```python
from build123d import *

# Parameters (mm, degrees)
EXTRUDE_1_DEPTH     = 1.45
SKETCH_3_R          = 3.5
EXTRUDE_2_DEPTH     = 2.02
SKETCH_4_R          = 2
CUT_EXTRUDE_1_DEPTH = 8.265654364
EXTRUDE_START       = -0.2
SKETCH_5_R          = 2
SKETCH_5_R_2        = 1.85
EXTRUDE_3_DEPTH     = 1.82
FILLET_1_R          = 0.75
FILLET_3_R          = 0.4


with BuildPart() as part:
    # 草图1 → 凸台-拉伸1 (new, symmetric)
    with BuildSketch(Plane(origin=(0, 0, 0), x_dir=(1, 0, 0), z_dir=(0, 1, 0))):
        Polygon((4.041451884, 0), (2.020725942, 3.5), (-2.020725942, 3.5), (-4.041451884, 0), (-2.020725942, -3.5), (2.020725942, -3.5), align=None)
    extrude(amount=EXTRUDE_1_DEPTH, both=True)

    # 草图3 → 凸台-拉伸2 (add)
    with BuildSketch(Plane(origin=(0, 1.45, 0), x_dir=(1, 0, 0), z_dir=(0, 1, 0))):
        with Locations(Location((0, 0, 0), (0, 0, 270))):
            Circle(SKETCH_3_R)
    extrude(amount=EXTRUDE_2_DEPTH)

    # 草图4 → 切除-拉伸1 (cut, through all)
    with BuildSketch(Plane(origin=(0, 3.47, 0), x_dir=(1, 0, 0), z_dir=(0, 1, 0))):
        with Locations(Location((0, 0, 0), (0, 0, 270))):
            Circle(SKETCH_4_R)
    extrude(amount=-CUT_EXTRUDE_1_DEPTH, mode=Mode.SUBTRACT)

    # 草图5 → 凸台-拉伸3 (add)
    with BuildSketch(Plane(origin=(0, 3.47, 0), x_dir=(1, 0, 0), z_dir=(0, 1, 0)).offset(EXTRUDE_START)):
        with Locations(Location((0, 0, 0), (0, 0, 270))):
            Circle(SKETCH_5_R)
        with Locations(Location((0, 0, 0), (0, 0, 270))):
            Circle(SKETCH_5_R_2, mode=Mode.SUBTRACT)
    extrude(amount=-EXTRUDE_3_DEPTH)

    # 圆角1
    # the kernel refuses this fillet: 0.75 mm, written as the material it takes off along each edge
    with BuildSketch(Plane(origin=(0, 3.47, 0), x_dir=(0, 0, 1), z_dir=(-1, 0, 0))) as fillet_1_piece_1:
        with BuildLine():
            CenterArc((3.5 - FILLET_1_R, -FILLET_1_R), FILLET_1_R, 0, 90)
            Line((3.5 - FILLET_1_R, 0), (3.5 - FILLET_1_R, FILLET_1_R * 0.02))
            Line((3.5 - FILLET_1_R, FILLET_1_R * 0.02), (3.5 + FILLET_1_R * 0.02, FILLET_1_R * 0.02))
            Line((3.5 + FILLET_1_R * 0.02, FILLET_1_R * 0.02), (3.5 + FILLET_1_R * 0.02, -FILLET_1_R))
            Line((3.5 + FILLET_1_R * 0.02, -FILLET_1_R), (3.5, -FILLET_1_R))
        make_face()
    revolve(axis=Axis((0, 3.47, 0), (0, 1, 0)), mode=Mode.SUBTRACT)
    with BuildSketch(Plane(origin=(0, 3.47, 0), x_dir=(0, 0, 1), z_dir=(-1, 0, 0))) as fillet_1_piece_2:
        with BuildLine():
            CenterArc((2.509901951, -0.75), FILLET_1_R, 90, 42.833428066)
            Line((2, -0.2), (1.989801961, -0.189))
            ThreePointArc((1.989801961, -0.189), (1.985, -0.1), (1.985, 0))
            Line((1.985, 0), (2, 0.015))
            Line((2, 0.015), (2.509901951, 0.015))
            Line((2.509901951, 0.015), (2.509901951, 0))
        make_face()
    revolve(axis=Axis((0, 3.47, 0), (0, 1, 0)), mode=Mode.SUBTRACT)

    # 草图6 → 切除-旋转1 (revolve, cut)
    with BuildSketch(Plane.XY):
        Polygon((-4.041451884, 1.45), (-4.041451884, 0.908548116), (-3.5, 1.45), align=None)
        Polygon((-4.041451884, -1.45), (-4.041451884, -0.908548116), (-3.5, -1.45), align=None)
    revolve(axis=Axis((0, -1000, 0), (0, 1, 0)), mode=Mode.SUBTRACT)

    # 圆角3
    fillet_3_edges = [part.edges().sort_by_distance(p)[0] for p in [
        (-4.041451884, 0, 0),
        (-2.020725942, 0, -3.5),
        (2.020725942, 0, -3.5),
        (4.041451884, 0, 0),
        (2.020725942, 0, 3.5),
        (-2.020725942, 0, 3.5),
    ]]
    fillet(fillet_3_edges, radius=FILLET_3_R)


solid = part.part
```
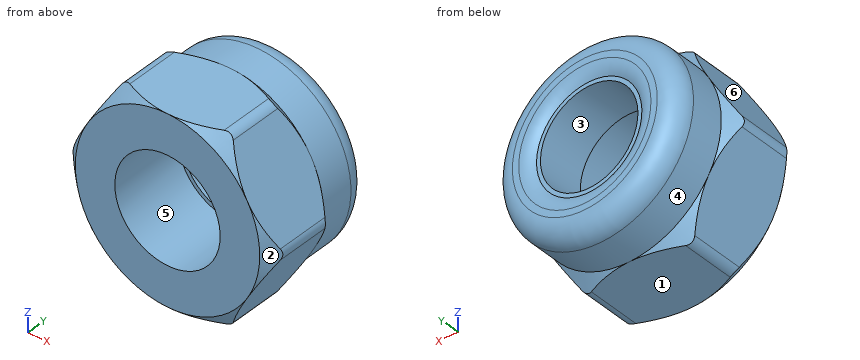
Work out the finished part from the listing and answer in its coordinate system (mm). Face numbers are marked on the shaded views. A direction names the side the tool comes from. Coordinates: 2 decimals unless noted, no trailing zeros. Loops run counter-clockwise (first coordinate to the right, second up) from the corner with the lowest first, then second, coordinate; pieces in that order, holes last. Notation, with made-up numbers: (9.5, 16.25) - (65.5, 16.25) arc R22 ccw to (65.5, 51.25) - close; hole circle Ø1 at (-7.75, 83.25). An arc over 180 degrees is marked (long way). Use a Markdown table: item, result.
Item 1: The mould has two halves that part along Z. Classify the marked faces 1, 2 and 3: +Z half, -Z half, draft (parallel to the pull), parting line (faces both ways), or undercut.
Evaluation:
| item | result |
|---|---|
| face 1 | -Z half |
| face 2 | parting line |
| face 3 | undercut |
Item 2: Consider probe 1 along X at (y, z) = (2.1, 0); probe 2 along X at (y, z) = (-0.6, 0); probe 3 along Z at (x, y) = (1, 0.75). Determine where each line is inside the solid, lowest interval first. Write a range as from..to.
Evaluation:
| item | result |
|---|---|
| probe 1 | x = -3.5..-1.85, 1.85..3.5 |
| probe 2 | x = -3.98..-2, 2..3.98 |
| probe 3 | z = -3.5..-1.73, 1.73..3.5 |
Item 3: For the marked faces 4, 5 and 6, determine the directions among +Z, -Z, +X, -X, +Y, -Y from which every point of the face is accessible in a straight line to the end or side of a thin tool.
Evaluation:
| item | result |
|---|---|
| face 4 | +Y |
| face 5 | -Y |
| face 6 | +Z, -X, +Y, -Y |
Item 4: Find section A-A, the plane z = 0. Determine the outline of the cut face in (x, y), and give its area (3 significant figures).
Evaluation:
| item | result |
|---|---|
| outline | (-3.98, -0.97) - (-3.5, -1.45) - (-2, -1.45) - (-2, 1.45) - (-1.85, 1.45) - (-1.85, 3.27) - (-2, 3.27) arc R0.75 ccw to (-2.51, 3.47) - (-2.75, 3.47) arc R0.75 ccw to (-3.5, 2.72) - (-3.5, 1.45) - (-3.98, 0.97) - close; (1.85, 1.45) - (2, 1.45) - (2, -1.45) - (3.5, -1.45) - (3.98, -0.97) - (3.98, 0.97) - (3.5, 1.45) - (3.5, 2.72) arc R0.75 ccw to (2.75, 3.47) - (2.51, 3.47) arc R0.75 ccw to (2, 3.27) - (1.85, 3.27) - close |
| area | 17.3 mm2 |
Item 5: Given pin 1 Ø2 at (x, z) = (1, -1) entering from +Y; pin 2 Ø1.5 at (x, y) = (3, 2.5) entering from -Z; pin 3 Ø1 at (y, z) = (-0.5, 2.5) entering from -X, each flat-ended and moving along its own axis, determine where each tip first touches the part or whether it passes through.
Evaluation:
| item | result |
|---|---|
| pin 1 | stops at y = 3.46 |
| pin 2 | stops at z = -2.68 |
| pin 3 | stops at x = -2.89 |
Item 6: Find section C-C, the plane y = 2.9. Determine the outline of the cut face in (x, z).
Evaluation:
| item | result |
|---|---|
| outline | circle Ø6.96 at (0, 0); hole circle Ø3.7 at (0, 0) |
Item 7: Find section B-B, the plane y = -0.3. Determine the outline of the cut face in (x, z), and give its area (3 significant figures).
Evaluation:
| item | result |
|---|---|
| outline | (-3.93, -0.2) - (-2.14, -3.3) arc R0.4 ccw to (-1.79, -3.5) - (1.79, -3.5) arc R0.4 ccw to (2.14, -3.3) - (3.93, -0.2) arc R0.4 ccw to (3.93, 0.2) - (2.14, 3.3) arc R0.4 ccw to (1.79, 3.5) - (-1.79, 3.5) arc R0.4 ccw to (-2.14, 3.3) - (-3.93, 0.2) arc R0.4 ccw to start; hole circle Ø4 at (0, 0) |
| area | 29.8 mm2 |
